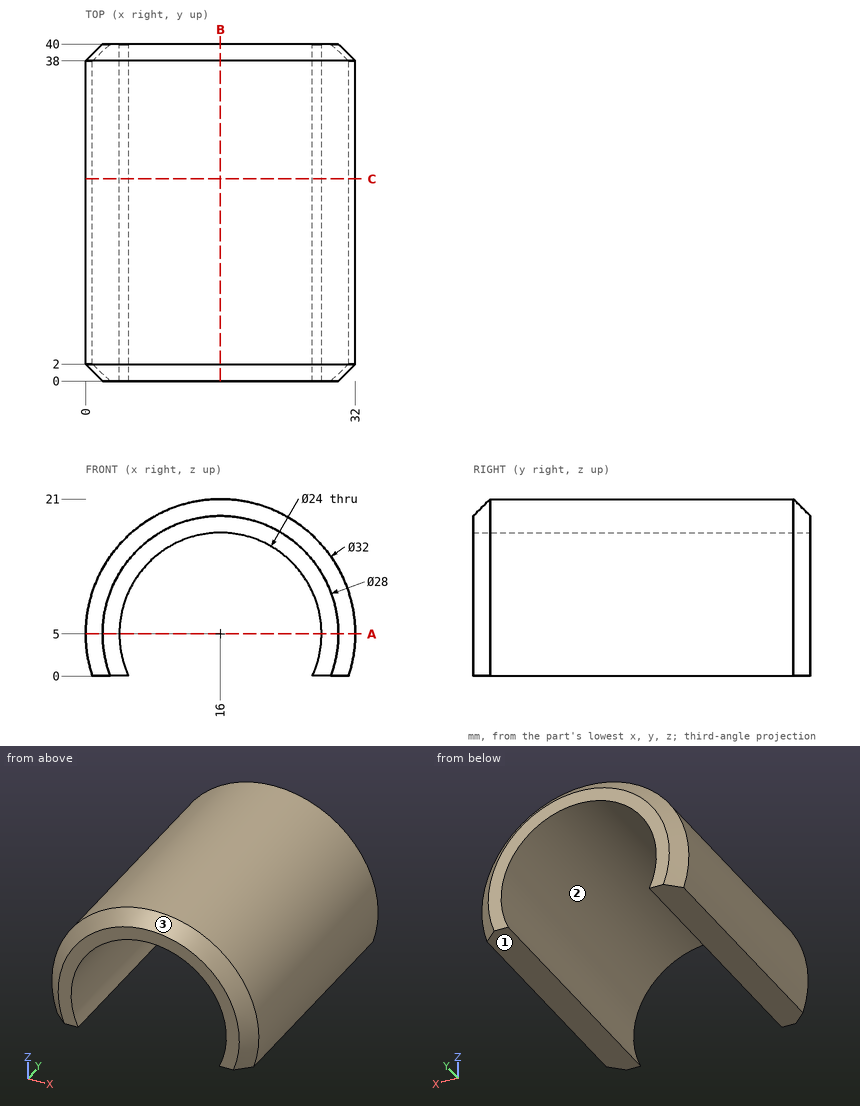
The figure shows three views and two pictorial views of one solid part (mm, origin at its lowest corner). Answer the questions. Give positions to 0.01 mm unless a question says otherwise; leave off trailing zeros. Order: outer loops, then holes, each group sorted by start corner. A loop starts at its lowest first (then second) coordinate and runs counter-clockwise, first axis right, second up. Notation, with made-up numbers: M -5.5,-22.5 L -1.5,-22.5 A17 ccw -1.5,2.5 Z; hole C 66,55.25 d7. An arc over 180 degrees is marked long. Return JSON: item names as keys, results as strings.
Q1. Each of these flat-tipped pins is pushed along its axis until it touches: pin 1 (3 mm diameter, centred on x = 19.5, z = 14.5, fed in from +Y); pin 2 (10 mm diameter, centred on x = 17, y = 34, fed in from -Z); pin 3 (8 mm diameter, centred on y = 36, z = 12, fed in from -X); pin 4 (8 mm diameter, centred on y = 30, z = 14, fed in from +X). Where does it stop, or does it pass through?
Answer below:
{"pin 1": "passes through", "pin 2": "stops at z = 15.39", "pin 3": "stops at x = 0.28", "pin 4": "stops at x = 31.2"}
Q2. Find section A-A, the plane z = 5. Write down the section's boundary in (x, y), and give its area (3 significant figures).
Answer below:
{"outline": "M 0,2 L 2,0 L 4,0 L 4,40 L 2,40 L 0,38 Z; M 28,0 L 30,0 L 32,2 L 32,38 L 30,40 L 28,40 Z", "area": "312 mm^2"}
Q3. The mould has two halves that part along Z. Classify the marked faces 1, 2 and 3: pulls with the +Z half, pulls with the -Z half, needs draft (parallel to the pull), parting line crosses it, or undercut.
Answer below:
{"face 1": "pulls with the -Z half", "face 2": "undercut", "face 3": "parting line crosses it"}
Q4. Find section B-B, the plane x = 16. Write down the section's boundary in (y, z).
Answer below:
{"outline": "M 0,17 L 40,17 L 40,19 L 38,21 L 2,21 L 0,19 Z"}
Q5. Find section C-C, the plane y = 24. Write down the section's boundary in (x, z), and give its area (3 significant figures).
Answer below:
{"outline": "M 0.8,0 L 5.09,0 A12 cw long 26.91,0 L 31.2,0 A16 ccw long Z", "area": "217 mm^2"}
Q6. Find the intervals of material crossed by line 1 along X through (y, z) = (27, 5); line 2 along Z through (x, y) = (16, 26); line 3 along X through (y, z) = (35, 15), in increasing order. Write a range as [from, to].
Answer below:
{"line 1": "x = [0, 4], [28, 32]", "line 2": "z = [17, 21]", "line 3": "x = [3.51, 9.37], [22.63, 28.49]"}
